from build123d import *

# Parameters (mm, degrees)
SKETCH1_W                                         = 180
SKETCH1_H                                         = 80
BOSS_EXTRUDE1_DEPTH                               = 10
SKETCH2_W                                         = 10
SKETCH2_H                                         = 10
BOSS_EXTRUDE2_DEPTH                               = 90
EXTRUDE_THIN1_DEPTH                               = 10
SKETCH4_W                                         = 10
SKETCH4_H                                         = 11.065155811
BOSS_EXTRUDE3_DEPTH                               = 80
RIB3_REACH                                        = 175.205
SKETCH5_WALL_W                                    = 376.694432762
SKETCH5_WALL_H                                    = 10
CUT_EXTRUDE1_START                                = -100
SKETCH6_R                                         = 3.175
CUT_EXTRUDE1_DEPTH                                = 100
CSK_FOR_1_FLAT_HEAD_MACHINE_SCREW_100_D           = 2.0574
CSK_FOR_1_FLAT_HEAD_MACHINE_SCREW_100_DEPTH       = 50
CSK_FOR_1_FLAT_HEAD_MACHINE_SCREW_100_CSINK_D     = 3.7084
CSK_FOR_1_FLAT_HEAD_MACHINE_SCREW_100_CSINK_ANGLE = 100
CSK_FOR_1_FLAT_HEAD_MACHINE_SCREW_100_TIP         = 0.618105319


with BuildPart() as part:
    # Sketch1 → Boss-Extrude1 (new body)
    with BuildSketch(Plane(origin=(0, 0, 0), x_dir=(1, 0, 0), z_dir=(0, 1, 0))):
        Polygon((100, 27.343827347), (100, 50), (-100, 50), (-100, 27.343827347), (-100, -27.343827347), (-100, -50), (100, -50), (100, -27.343827347), align=None)
        Rectangle(SKETCH1_W, SKETCH1_H, mode=Mode.SUBTRACT)
    extrude(amount=BOSS_EXTRUDE1_DEPTH)

    # Sketch2 → Boss-Extrude2 (add)
    with BuildSketch(Plane(origin=(0, 10, 0), x_dir=(1, 0, 0), z_dir=(0, 1, 0))):
        with Locations((95, -45)):
            Rectangle(SKETCH2_W, SKETCH2_H)
        with Locations((95, 45)):
            Rectangle(SKETCH2_W, SKETCH2_H)
    extrude(amount=BOSS_EXTRUDE2_DEPTH)

    # Sketch3 → Extrude-Thin1 (add)
    with BuildSketch(Plane.XY.offset(50)):
        Polygon((-100, 10), (90, 100), (94.280863447, 90.962621611), (-95.719136553, 0.962621611), align=None)
    extrude_thin1 = extrude(amount=-EXTRUDE_THIN1_DEPTH)

    # Mirror1: Extrude-Thin1 across plane
    add(extrude_thin1.mirror(Plane.XY))

    # Sketch4 → Boss-Extrude3 (add)
    with BuildSketch(Plane.XY.offset(-40)):
        with Locations((95, 94.467422094)):
            Rectangle(SKETCH4_W, SKETCH4_H)
    extrude(amount=BOSS_EXTRUDE3_DEPTH)

    # Sketch5 wall → Rib3 (add, up to next)
    with BuildSketch(Plane(origin=(80, 20, 50), x_dir=(-0.707106781187, -0.707106781187, 0), z_dir=(0.707106781187, -0.707106781187, 0)), mode=Mode.PRIVATE) as rib3_sk1:
        with Locations((0, 5)):
            Rectangle(SKETCH5_WALL_W, SKETCH5_WALL_H)
    rib3_tool1 = extrude(rib3_sk1.sketch, amount=RIB3_REACH, mode=Mode.PRIVATE) - part.part
    rib3 = rib3_tool1.solids().sort_by_distance((80, 20, 50))[0]
    add(rib3)

    # Mirror2: Rib3 across plane
    add(rib3.mirror(Plane.XY))

    # Sketch6 → Cut-Extrude1 (cut)
    with BuildSketch(Plane.XY.offset(50).offset(CUT_EXTRUDE1_START)):
        with Locations((84.882990755, 15.483266945)):
            Circle(SKETCH6_R)
    extrude(amount=CUT_EXTRUDE1_DEPTH, mode=Mode.SUBTRACT)

    # CSK for #1 Flat Head Machine Screw (100)1
    with Locations(Plane(origin=(0, 10, 0), x_dir=(1, 0, 0), z_dir=(0, 1, 0))):
        with Locations((-94.584598499, -30), (-94.584598499, 30), (94.978129644, 30), (94.978129644, -30)):
            CounterSinkHole(CSK_FOR_1_FLAT_HEAD_MACHINE_SCREW_100_D / 2, CSK_FOR_1_FLAT_HEAD_MACHINE_SCREW_100_CSINK_D / 2, depth=CSK_FOR_1_FLAT_HEAD_MACHINE_SCREW_100_DEPTH, counter_sink_angle=CSK_FOR_1_FLAT_HEAD_MACHINE_SCREW_100_CSINK_ANGLE)
            with Locations((0, 0, -(CSK_FOR_1_FLAT_HEAD_MACHINE_SCREW_100_DEPTH + CSK_FOR_1_FLAT_HEAD_MACHINE_SCREW_100_TIP / 2))):  # 118° drill point
                Cone(0, CSK_FOR_1_FLAT_HEAD_MACHINE_SCREW_100_D / 2, CSK_FOR_1_FLAT_HEAD_MACHINE_SCREW_100_TIP, mode=Mode.SUBTRACT)


solid = part.part
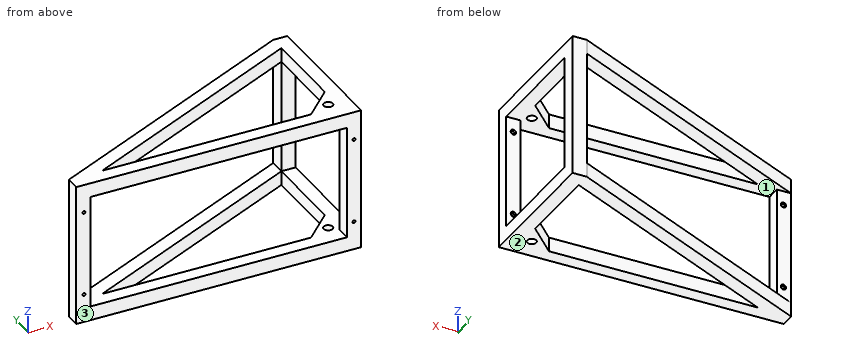
CAD build for the part. Positions are in the model's coordinates, mm. Face numbers are marked on the shaded views. Round coordinates to 2 decimals unless told otherwise and drop trailing zeros. Order: outer loops, then holes, each group sorted by start corner. A loop starts at its lowest first (then second) coordinate and runs counter-clockwise, first axis right, second up. Notation, with made-up numbers: (73, -29) - (98, -29) arc R28 ccw to (98, -11) - close; hole circle Ø11 at (33.25, 14.5). An arc over 180 degrees is marked (long way). Return JSON: item names as keys, results as strings.
(1) Cut at B-B (y = 23). Give the cut face in (x, z).
Answer key:
{"outline": "(-72.56, -50) - (-49.2, -50) - (-49.2, -40) - (-72.56, -40) - close; (-72.56, 40) - (-49.2, 40) - (-49.2, 50) - (-72.56, 50) - close; (83, -50) - (100, -50) - (100, -40) - (83, -40) - close; (83, 40) - (100, 40) - (100, 50) - (83, 50) - close"}
(2) Wall check: probe 1 along X at (y, z) = (4, -30); probe 2 along Z at (x, y) = (-83, 8); probe 3 along X at (y, z) = (7.5, -2). Give the ranges that are in metal, low to high. Write a range as from..to.
Answer key:
{"probe 1": "x = -100..-95.61, -93.56..-90, 90..93.95, 96.01..100", "probe 2": "z = -50..-40, 40..50", "probe 3": "x = -100..-90, 90..100"}
(3) Cut at C-C (x = -46.5). Give the cut face in (y, z).
Answer key:
{"outline": "(0, -50) - (10, -50) - (10, -40) - (0, -40) - close; (0, 40) - (10, 40) - (10, 50) - (0, 50) - close; (24.28, -50) - (35.34, -50) - (35.34, -40) - (24.28, -40) - close; (24.28, 40) - (35.34, 40) - (35.34, 50) - (24.28, 50) - close"}
(4) Cut at A-A (z = 21). Give the cut face in (x, y), then the cut area to 3 significant figures.
Answer key:
{"outline": "(-100, 0) - (-90, 0) - (-90, 10) - (-100, 10) - close; (90, 0) - (100, 0) - (100, 10) - (90, 10) - close; (90, 88.93) - (100, 88.93) - (100, 100) - (90, 100) - close", "area": "311 mm^2"}
(5) Cut at D-D (y = 92). Give the cut face in (x, z).
Answer key:
{"outline": "(73.11, -50) - (100, -50) - (100, 50) - (73.11, 50) - (73.11, 40) - (90, 40) - (90, -40) - (73.11, -40) - close"}
(6) Pull direction Y, two halves, no side cores. Call the marked faces 1, 2 and 3: +Y half, -Y half, draft (parallel to the pull), parting line (faces both ways), or undercut.
Answer key:
{"face 1": "undercut", "face 2": "draft", "face 3": "-Y half"}
(7) Pin check, flat tips, straight feed: pin 1 Ø5 at (x, y) = (84.88, 15.48) entering from -Z; pin 2 Ø11 at (y, z) = (73, -45) entering from -X; pin 3 Ø5 at (x, z) = (21, -44) entering from +Y; pin 4 Ø1.2 at (x, z) = (94.98, 30) entering from -Y. Stop position of each tip, or through.
Answer key:
{"pin 1": "passes through", "pin 2": "stops at x = 21.39", "pin 3": "stops at y = 68.5", "pin 4": "stops at y = 88.93"}
